Source: CAD feature listing. Evaluate the final solid. Frame: model axes, mm. A direction names the side the tool comes from. Coordinates: 2 decimals unless noted, no trailing zeros. Order: outer loops, then holes, each group sorted by start corner. A loop starts at its lowest first (then second) coordinate and runs counter-clockwise, first axis right, second up. Notation, with made-up numbers: (-18, 54) -> (-14, 54) arc R17 cw to (-14, 84) -> close; hole circle Ø6 at (23.5, 56). An arc over 180 degrees is marked (long way). Write item = value, one per line. Start each with the question number.
Item 1: Contact query for flat-ended pins moving along their axis: pin 1 (1.5 mm diameter, centred on x = -2.5, y = 7.5, fed in from +Z); pin 2 (4 mm diameter, centred on x = 0, y = 0, fed in from -Z); pin 3 (6 mm diameter, centred on x = -0.5, y = 5.5, fed in from +Z); pin 4 (3 mm diameter, centred on x = 0.5, y = -5, fed in from +Z). Output: stop coordinate, or through.
Item 2: Mould query, pull axis X, two halves, no side actions, for faces 1 (the flat face through (13, -2, 4)), 2 (the flat face through (-6, 0, 7)), 3 (the flat face through (-3, -6, 7)). Classes: released by +X, released by -X, zero draft, split by the parting line, or undercut.
Item 3: Section query A-A (z = 6.75). Output: boundary loops of the cut face in (x, y).
Item 4: Section query C-C (y = 0). Output: boundary loops of the cut face in (x, z).
Item 5: Section query D-D (z = 4.25). Output: boundary loops of the cut face in (x, y), then the cut area to 3 significant figures.
Item 6: Ray query, line 1 along X through (y, z) = (-5.25, 4.5); line 2 along Y through (x, z) = (0, 4.7); line 3 along X through (y, z) = (-9.25, 4.75). Return the intervals inside material, ascending. Write a range as [from, to].
Item 7: Set-up query: faces 4 (the cylindrical face through (-12.14, 12.1, 3.16)), 5 (the cylindrical face through (-7.9, -10, 3.8)), 6 (the flat face through (3, -6, 7)). Return all of +Z, -Z, +X, -X, +Y, -Y with unobstructed straight access to the full face (end or side cutting, diameter ignored); none if empty.
Item 8: Section query B-B (x = 7.9). Output: boundary loops of the cut face in (y, z), then the cut area to 3 significant figures.
```python
from build123d import *

# Parameters (mm, degrees)
SKETCH_1_W               = 26
SKETCH_1_H               = 26
EXTRUDE_1_DEPTH          = 8
CUT_EXTRUDE_1_DEPTH      = 21.049937656
CUT_EXTRUDE_1_DEPTH_BACK = 21.049937656
SKETCH_2_OUTSIDE_W       = 17.526
SKETCH_2_OUTSIDE_H       = 35.526
HOLE_WIZARD_M3_1_D       = 3.2
SKETCH_4_OUTSIDE_W       = 17.526
SKETCH_4_OUTSIDE_H       = 35.526
SKETCH_4_OUTSIDE_W_2     = 6
SKETCH_4_OUTSIDE_H_2     = 26
CUT_EXTRUDE_2_DEPTH      = 3
FILLET_1_R               = 3


with BuildPart() as part:
    # ｽｹｯﾁ1 → ﾎﾞｽ - 押し出し1 (new body)
    with BuildSketch(Plane.XY):
        Rectangle(SKETCH_1_W, SKETCH_1_H)
        with BuildLine():
            Line((-6.3, 8.4), (-6.3, -8.4))
            ThreePointArc((-6.3, -8.4), (-7.9, -10), (-9.5, -8.4))
            Line((-9.5, -8.4), (-9.5, 8.4))
            ThreePointArc((-9.5, 8.4), (-7.9, 10), (-6.3, 8.4))
        make_face(mode=Mode.SUBTRACT)
        with BuildLine():
            Line((9.5, 8.4), (9.5, -8.4))
            ThreePointArc((9.5, -8.4), (7.9, -10), (6.3, -8.4))
            Line((6.3, -8.4), (6.3, 8.4))
            ThreePointArc((6.3, 8.4), (7.9, 10), (9.5, 8.4))
        make_face(mode=Mode.SUBTRACT)
    extrude(amount=EXTRUDE_1_DEPTH)

    # ｽｹｯﾁ2 outside → ｶｯﾄ - 押し出し1 (cut, two sides: drawn at the far end of the back side and taken through both)
    with BuildSketch(Plane(origin=(0, 0, 0), x_dir=(0, 0, -1), z_dir=(1, 0, 0)).offset(-CUT_EXTRUDE_1_DEPTH_BACK)):
        with Locations((-4, 0)):
            Rectangle(SKETCH_2_OUTSIDE_W, SKETCH_2_OUTSIDE_H)
        Polygon((0, -13), (-8, -13), (-6, 13), (0, 13), align=None, mode=Mode.SUBTRACT)
    extrude(amount=CUT_EXTRUDE_1_DEPTH + CUT_EXTRUDE_1_DEPTH_BACK, mode=Mode.SUBTRACT)

    # M3 すきま穴1 (through all)
    with Locations(Plane(origin=(0, 0, 0), x_dir=(-1, 0, 0), z_dir=(0, 0, -1))):
        with Locations((0, 0)):
            Hole(HOLE_WIZARD_M3_1_D / 2)

    # ｽｹｯﾁ4 outside → ｶｯﾄ - 押し出し2 (cut, symmetric)
    with BuildSketch(Plane(origin=(0, 0, 0), x_dir=(0, 0, -1), z_dir=(1, 0, 0))):
        with Locations((-4, 0)):
            Rectangle(SKETCH_4_OUTSIDE_W, SKETCH_4_OUTSIDE_H)
        with Locations((-3, 0)):
            Rectangle(SKETCH_4_OUTSIDE_W_2, SKETCH_4_OUTSIDE_H_2, mode=Mode.SUBTRACT)
    extrude(amount=CUT_EXTRUDE_2_DEPTH, both=True, mode=Mode.SUBTRACT)

    # ﾌｨﾚｯﾄ1
    fillet_1_edges = [part.edges().sort_by_distance(p)[0] for p in [
        (-13, 13, 3),
        (13, 13, 3),
    ]]
    fillet(fillet_1_edges, radius=FILLET_1_R)


solid = part.part
```
Computed:
q1.pin_1 = 6.47
q1.pin_2 = 0
q1.pin_3 = 6.7
q1.pin_4 = 6
q2.face_1 = released by +X
q2.face_2 = zero draft
q2.face_3 = undercut
q3.outline = (-13, -13) -> (-3, -13) -> (-3, 3.25) -> (-6.3, 3.25) -> (-6.3, -8.4) arc R1.6 cw to (-9.5, -8.4) -> (-9.5, 3.25) -> (-13, 3.25) -> close; (3, -13) -> (13, -13) -> (13, 3.25) -> (9.5, 3.25) -> (9.5, -8.4) arc R1.6 cw to (6.3, -8.4) -> (6.3, 3.25) -> (3, 3.25) -> close
q4.outline = (-13, 0) -> (-9.5, 0) -> (-9.5, 7) -> (-13, 7) -> close; (-6.3, 0) -> (-1.6, 0) -> (-1.6, 6) -> (-3, 6) -> (-3, 7) -> (-6.3, 7) -> close; (1.6, 0) -> (6.3, 0) -> (6.3, 7) -> (3, 7) -> (3, 6) -> (1.6, 6) -> close; (9.5, 0) -> (13, 0) -> (13, 7) -> (9.5, 7) -> close
q5.outline = (-13, -13) -> (13, -13) -> (13, 10) arc R3 ccw to (10, 13) -> (-10, 13) arc R3 ccw to (-13, 10) -> close; hole (-9.5, -8.4) arc R1.6 ccw to (-6.3, -8.4) -> (-6.3, 8.4) arc R1.6 ccw to (-9.5, 8.4) -> close; hole circle Ø3.2 at (0, 0); hole (6.3, -8.4) arc R1.6 ccw to (9.5, -8.4) -> (9.5, 8.4) arc R1.6 ccw to (6.3, 8.4) -> close
q5.area = 540 mm^2
q6.line_1 = [-13, -9.5], [-6.3, 6.3], [9.5, 13]
q6.line_2 = [-13, -1.6], [1.6, 13]
q6.line_3 = [-13, -9.26], [-6.54, 6.54], [9.26, 13]
q7.face_4 = +Z, -Z, -X, +Y
q7.face_5 = +Z, -Z
q7.face_6 = +Z, +Y, -Y
q8.outline = (-13, 0) -> (-10, 0) -> (-10, 7.77) -> (-13, 8) -> close; (10, 0) -> (13, 0) -> (13, 6) -> (10, 6.23) -> close
q8.area = 42.0 mm^2
